Part print with two shaded views. Sizes in mm from the minimum x, y, z corner. Round coordinates to 2 decimals unless told otherwise and drop trailing zeros. Order: outer loops, then holes, each group sorted by start corner. A loop starts at its lowest first (then second) coordinate and runs counter-clockwise, first axis right, second up. Notation, with made-up numbers: M -10,59 L 18,59 A25 ccw 18,96 Z; hole C 1.25,-7.75 d11. An arc over 180 degrees is marked long. One line per question, with ' | ' between items.
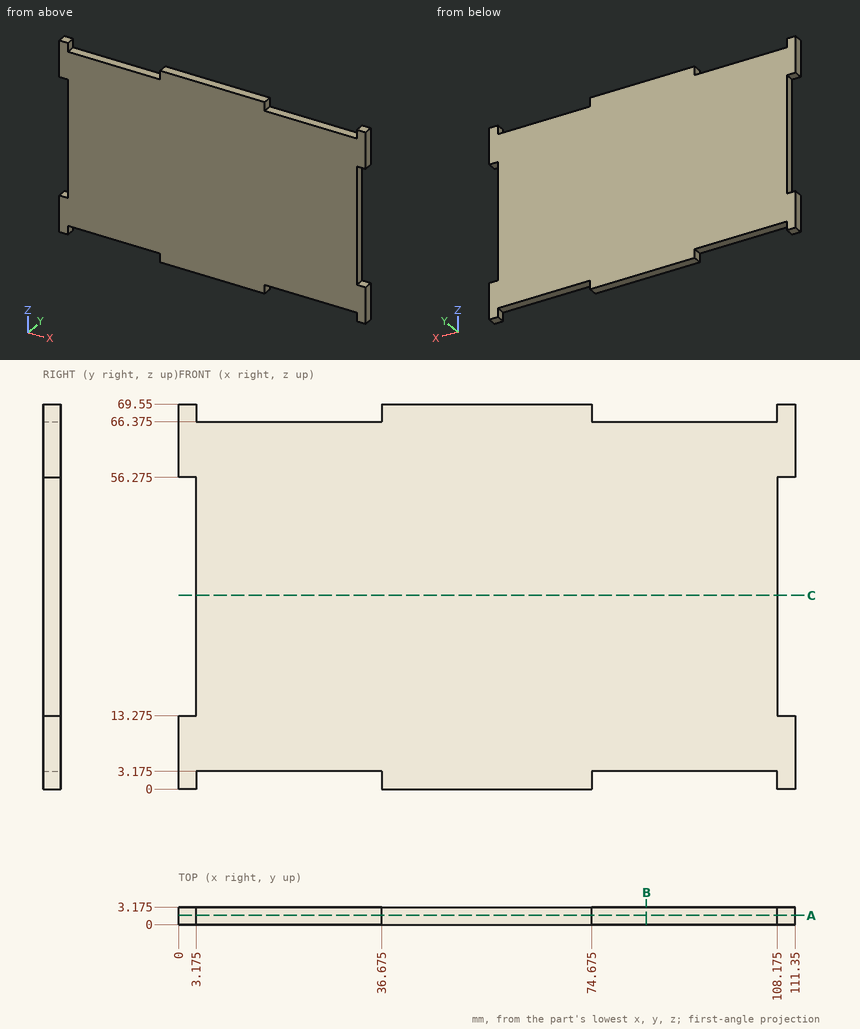
1) Saw through at C-C (z = 35). List the corners of the cut face in (x, y) (3 decimals), plus the area to 3 significant figures.
The answers:
outline: M 3.175,0 L 108.175,0 L 108.175,3.175 L 3.175,3.175 Z | area: 333 mm²
2) Drop flat-ended pins along their axis: pin 1 (1.6 mm diameter, centred on x = 88.5, y = 2, fed in from +Z) (3 decimals); pin 2 (1 mm diameter, centred on y = 1, z = 68.5, fed in from -X); pin 3 (1.5 mm diameter, centred on y = 1.5, z = 22, fed in from -X) (3 decimals). Give the stop position or say it passes through.
The answers:
pin 1: stops at z = 66.375 | pin 2: stops at x = 0 | pin 3: stops at x = 3.175
3) Saw through at B-B (x = 84.5). List the corners of the cut face in (y, z) (3 decimals), plus the area to 3 significant figures.
The answers:
outline: M 0,3.175 L 3.175,3.175 L 3.175,66.375 L 0,66.375 Z | area: 201 mm²
4) Probe line 1 (Z direction, x = 34, y = 0.7) (3 decimals); line 2 (X direction, y = 2.3, z = 41.5) (3 decimals). List the from-to ranges inside material, lowest first. Write a range as [from, to].
The answers:
line 1: z = [3.175, 66.375] | line 2: x = [3.175, 108.175]
5) Saw through at A-A (y = 1.65). List the corners of the cut face in (x, z) (3 decimals).
The answers:
outline: M 0,0 L 3.175,0 L 3.175,3.175 L 36.675,3.175 L 36.675,0 L 74.675,0 L 74.675,3.175 L 108.175,3.175 L 108.175,0 L 111.35,0 L 111.35,13.275 L 108.175,13.275 L 108.175,56.275 L 111.35,56.275 L 111.35,69.55 L 108.175,69.55 L 108.175,66.375 L 74.675,66.375 L 74.675,69.55 L 36.675,69.55 L 36.675,66.375 L 3.175,66.375 L 3.175,69.55 L 0,69.55 L 0,56.275 L 3.175,56.275 L 3.175,13.275 L 0,13.275 Z
